```python
from build123d import *

# Parameters (mm, degrees)
SKETCH_W      = 75
SKETCH_H      = 50
SKETCH_R      = 3.5
SKETCH_R_2    = 3.75
SKETCH_R_3    = 1.25
PAD_DEPTH     = 2
SKETCH001_W   = 75
SKETCH001_H   = 50
SKETCH001_W_2 = 71
SKETCH001_H_2 = 46
PAD001_DEPTH  = 20
SKETCH002_W   = 50
SKETCH002_H   = 15
POCKET_DEPTH  = 25.001


with BuildPart() as part:
    # Sketch → Pad (new body)
    with BuildSketch(Plane.XY):
        Rectangle(SKETCH_W, SKETCH_H)
        with Locations((0, -15)):
            Circle(SKETCH_R, mode=Mode.SUBTRACT)
        with Locations((25, -15)):
            Circle(SKETCH_R_2, mode=Mode.SUBTRACT)
        with Locations((-25, -15)):
            Circle(SKETCH_R_2, mode=Mode.SUBTRACT)
        with Locations((-11.75, 20)):
            Circle(SKETCH_R_3, mode=Mode.SUBTRACT)
        with Locations((-11.75, -3.8)):
            Circle(SKETCH_R_3, mode=Mode.SUBTRACT)
        with Locations((11.75, -3.8)):
            Circle(SKETCH_R_3, mode=Mode.SUBTRACT)
        with Locations((11.75, 20)):
            Circle(SKETCH_R_3, mode=Mode.SUBTRACT)
        Polygon((-12.5, 18.25), (-12.5, 0.25), (-6.25, 0.25), (-6.25, -4.75), (6.25, -4.75), (6.25, 0.25), (12.5, 0.25), (12.5, 18.25), (5, 18.25), (5, 22.25), (-5, 22.25), (-5, 18.25), align=None, mode=Mode.SUBTRACT)
    extrude(amount=-PAD_DEPTH)

    # Sketch001 → Pad001 (join)
    with BuildSketch(Plane.XY):
        Rectangle(SKETCH001_W, SKETCH001_H)
        Rectangle(SKETCH001_W_2, SKETCH001_H_2, mode=Mode.SUBTRACT)
    extrude(amount=PAD001_DEPTH)

    # Sketch002 → Pocket (cut, through all)
    with BuildSketch(Plane.XZ):
        with Locations((0, 12.5)):
            Rectangle(SKETCH002_W, SKETCH002_H)
    extrude(amount=-POCKET_DEPTH, mode=Mode.SUBTRACT)


solid = part.part
```
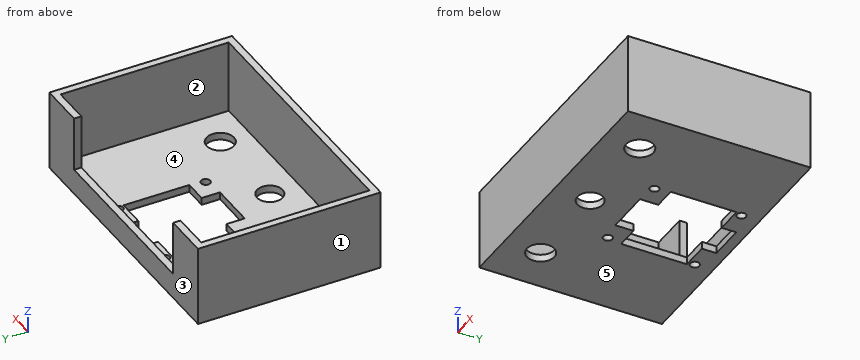
The listing builds one solid part. Answer for the finished solid, in the listing's coordinates (mm). Face numbers are marked on the shaded views. A direction names the side the tool comes from. Coordinates: 2 decimals unless noted, no trailing zeros. Write each loop counter-clockwise with the first axis right and the second up, starting at its lowest first coordinate (ties: lowest second). Pieces come first, ordered by that corner, then holes. Notation, with made-up numbers: (48, 4.5) -> (62, 4.5) arc R28 cw to (62, 42.5) -> close; hole circle Ø11 at (12, 5). An arc over 180 degrees is marked (long way). Write each question's results on one line, items separated by ' | '. Start each with the question number.
1) Straight lines are drawn through the part: probe 1 along Y at (x, z) = (0, -0.9); probe 2 along Y at (x, z) = (17, 4.75); probe 3 along X at (y, z) = (-16, 16). For each, find the intervals that lie inside material, in ascending order.
2) A cutting plane is placed at A-A (y = -15). Determine the outline of the cut face in (x, z), then the cut area to 3 significant figures.
3) A cutting plane is placed at D-D (x = 11.75). Determine the outline of the cut face in (y, z), then the cut area to 3 significant figures.
4) A tool of negligible diameter and unlimited length cuts with its end or side. For the marked faces 1 and 2, from which of +Z, -Z, +X, -X, +Y, -Y can it reach the whole face along a straight path? Write none if from no direction.
5) Flat-ended cylindrical pins translate along their axes: pin 1 Ø9 at (x, y) = (0, -15) entering from -Z; pin 2 Ø12 at (x, y) = (6, 8) entering from +Z; pin 3 Ø3 at (x, y) = (-11.75, 20) entering from +Z. Find the tip coordinate at first contact, or state that the pin passes through.
6) For a pull along Y with two mould halves and no side action, classify the marked faces 3, 4 and 5 as +Y half, -Y half, draft (parallel to the pull), parting line (faces both ways), or undercut.
7) A cutting plane is placed at B-B (x = 23.5). Determine the outline of the cut face in (y, z), then the cut area to 3 significant figures.
8) A cutting plane is placed at C-C (y = 14). Determine the outline of the cut face in (x, z), then the cut area to 3 significant figures.
Values follow:
1) probe 1: -25 to -18.5, -11.5 to -4.75, 22.25 to 25 | probe 2: -25 to -23, 23 to 25 | probe 3: -37.5 to -35.5, 35.5 to 37.5
2) outline: (-37.5, -2) -> (-28.75, -2) -> (-28.75, 0) -> (-35.5, 0) -> (-35.5, 20) -> (-37.5, 20) -> close; (-21.25, -2) -> (-3.5, -2) -> (-3.5, 0) -> (-21.25, 0) -> close; (3.5, -2) -> (21.25, -2) -> (21.25, 0) -> (3.5, 0) -> close; (28.75, -2) -> (37.5, -2) -> (37.5, 20) -> (35.5, 20) -> (35.5, 0) -> (28.75, 0) -> close | area: 186 mm²
3) outline: (-25, -2) -> (-5.05, -2) -> (-5.05, 0) -> (-23, 0) -> (-23, 20) -> (-25, 20) -> close; (-2.55, -2) -> (0.25, -2) -> (0.25, 0) -> (-2.55, 0) -> close; (18.25, -2) -> (18.75, -2) -> (18.75, 0) -> (18.25, 0) -> close; (21.25, -2) -> (25, -2) -> (25, 5) -> (23, 5) -> (23, 0) -> (21.25, 0) -> close | area: 104 mm²
4) face 1: +Z, -Z, -X, +Y, -Y | face 2: +Z
5) pin 1: z = -2 | pin 2: through | pin 3: z = 0
6) face 3: +Y half | face 4: undercut | face 5: draft
7) outline: (-25, -2) -> (-18.44, -2) -> (-18.44, 0) -> (-23, 0) -> (-23, 20) -> (-25, 20) -> close; (-11.56, -2) -> (25, -2) -> (25, 5) -> (23, 5) -> (23, 0) -> (-11.56, 0) -> close | area: 136 mm²
8) outline: (-37.5, -2) -> (-12.5, -2) -> (-12.5, 0) -> (-35.5, 0) -> (-35.5, 20) -> (-37.5, 20) -> close; (12.5, -2) -> (37.5, -2) -> (37.5, 20) -> (35.5, 20) -> (35.5, 0) -> (12.5, 0) -> close | area: 180 mm²
